Drawing for the job (mm, zero at the part's lowest x, y, z). A direction names the side the tool comes from. Round coordinates to 2 decimals unless told otherwise and drop trailing zeros. Write each loop counter-clockwise with the first axis right and the second up, starting at its lowest first coordinate (ties: lowest second). Pieces come first, ordered by that corner, then holes.
Item 1: Band-saw the part on D-D, the plane z = 223.5. Write the cut outline in (x, y), then the cut area to 3 significant figures.
Item 2: 3-axis set-ups, long thin cutter, end or side, ignore diameter. For the marked faces 1, 2 and 3: which of +Z, -Z, +X, -X, +Y, -Y reach the whole face in a straight line?
Item 3: Band-saw the part on C-C, the plane x = 95. Write the cut outline in (y, z), then the cut area to 3 significant figures.
Item 4: Band-saw the part on B-B, the plane z = 144.5. Write the cut outline in (x, y), then the cut area to 3 significant figures.
Item 5: Drop flat-ended pins along their axis: pin 1 Ø2 at (x, y) = (40, 79) entering from -Z; pin 2 Ø5 at (x, z) = (108, 261.5) entering from -Y; pin 3 Ø1.5 at (y, z) = (61.5, 242.5) entering from -X. Give the stop position or say it passes through.
Item 6: Band-saw the part on A-A, the plane y = 48.5. Write the cut outline in (x, z).
Item 7: Wall check: probe 1 along Z at (x, y) = (65, 16.5); probe 2 along X at (y, z) = (26, 138.5); probe 3 along Y at (x, z) = (74, 263.5). Give the ranges that are in metal, low to high.
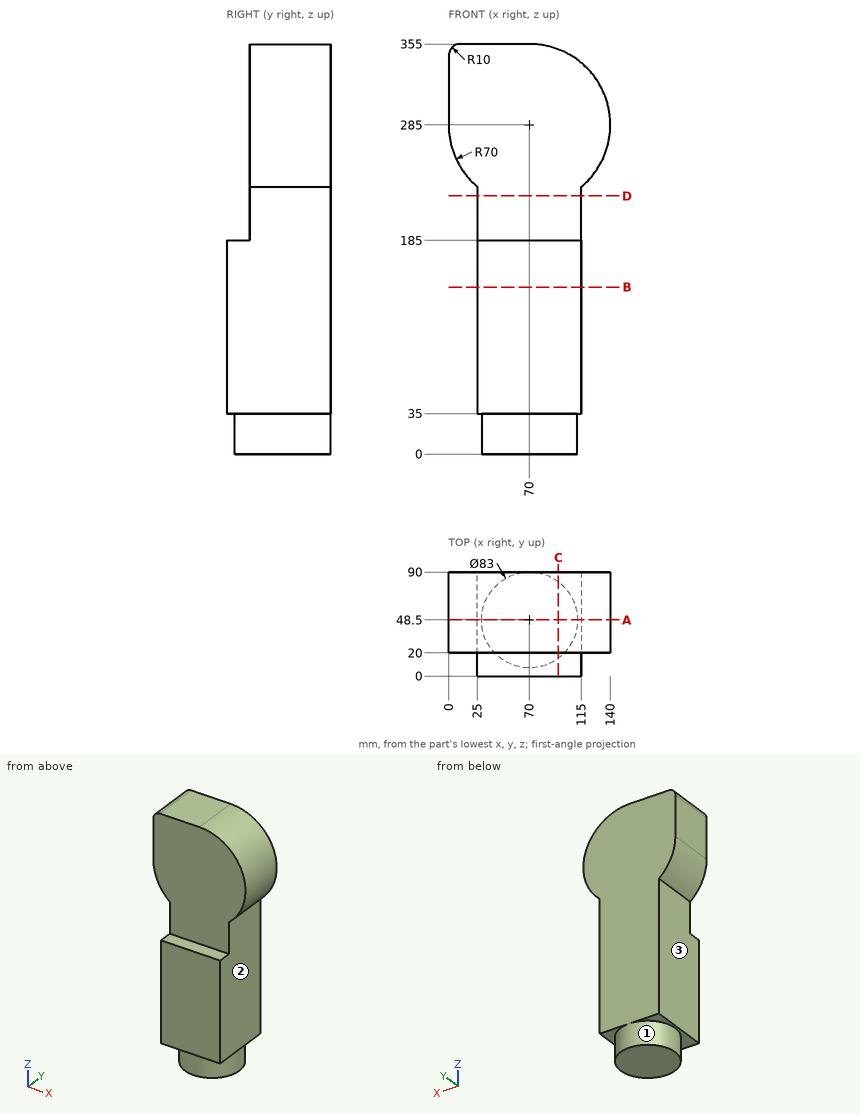
Results:
1. outline: (25, 20) - (115, 20) - (115, 90) - (25, 90) - close
1. area: 6,300 mm2
2. face 1: -Z
2. face 2: -Z, +X, +Y, -Y
2. face 3: -Z, -X, +Y, -Y
3. outline: (0, 35) - (15.38, 35) - (15.38, 0) - (81.62, 0) - (81.62, 35) - (90, 35) - (90, 350.38) - (20, 350.38) - (20, 185) - (0, 185) - close
3. area: 27,400 mm2
4. outline: (25, 0) - (115, 0) - (115, 90) - (25, 90) - close
4. area: 8,100 mm2
5. pin 1: stops at z = 35
5. pin 2: stops at y = 20
5. pin 3: stops at x = 13.81
6. outline: (0, 285) arc R70 ccw to (25, 231.38) - (25, 35) - (28.5, 35) - (28.5, 0) - (111.5, 0) - (111.5, 35) - (115, 35) - (115, 231.38) arc R70 ccw to (70, 355) - (10, 355) arc R10 ccw to (0, 345) - close
7. probe 1: z = 0 to 185
7. probe 2: x = 25 to 115
7. probe 3: y = 20 to 90
